```python
from build123d import *

# Parameters (mm, degrees)
IZIM1_R                     = 65
IZIM1_W                     = 20
IZIM1_H                     = 5
Y_KSEKLIK_EKSTR_ZYON1_DEPTH = 3
Y_KSEKLIK_EKSTR_ZYON2_START = 2
IZIM2_R                     = 65
Y_KSEKLIK_EKSTR_ZYON2_DEPTH = 2
SKETCH1_OUTSIDE_W           = 168.784
SKETCH1_OUTSIDE_H           = 168.784
CUT_EXTRUDE1_DEPTH          = 10


with BuildPart() as part:
    # Çizim1 → Yükseklik-Ekstrüzyon1 (new body)
    with BuildSketch(Plane.XY):
        Circle(IZIM1_R)
        Polygon((6.197521384, -35.508725619), (5.430030224, -40.449470231), (25.193008671, -43.519434871), (25.960499832, -38.578690259), (16.079010608, -37.043707939), align=None, mode=Mode.SUBTRACT)
        Polygon((8.806991329, -18.710193939), (8.039500168, -23.650938551), (17.920989392, -25.185920871), (27.802478616, -26.720903191), (28.569969776, -21.780158579), align=None, mode=Mode.SUBTRACT)
        with Locations((-33, -8.5)):
            Rectangle(IZIM1_W, IZIM1_H, mode=Mode.SUBTRACT)
        with Locations((-33, 8.5)):
            Rectangle(IZIM1_W, IZIM1_H, mode=Mode.SUBTRACT)
        Polygon((17.920989392, 25.185920871), (8.039500168, 23.650938551), (8.806991329, 18.710193939), (28.569969776, 21.780158579), (27.802478616, 26.720903191), align=None, mode=Mode.SUBTRACT)
        Polygon((16.079010608, 37.043707939), (25.960499832, 38.578690259), (25.193008671, 43.519434871), (5.430030224, 40.449470231), (6.197521384, 35.508725619), align=None, mode=Mode.SUBTRACT)
    extrude(amount=Y_KSEKLIK_EKSTR_ZYON1_DEPTH)

    # Çizim2 → Yükseklik-Ekstrüzyon2 (add)
    with BuildSketch(Plane(origin=(0, 0, 0), x_dir=(-1, 0, 0), z_dir=(0, 0, -1)).offset(Y_KSEKLIK_EKSTR_ZYON2_START)):
        Circle(IZIM2_R)
    extrude(amount=-Y_KSEKLIK_EKSTR_ZYON2_DEPTH)

    # Sketch1 outside → Cut-Extrude1 (cut)
    with BuildSketch(Plane.XY.offset(3)):
        Rectangle(SKETCH1_OUTSIDE_W, SKETCH1_OUTSIDE_H)
        with BuildLine():
            Line((-46.208680474, -21.225709885), (3.791319526, -52.34052429))
            ThreePointArc((3.791319526, -52.34052429), (29.140489861, -52.969070419), (42, -31.114814405))
            Line((42, -31.114814405), (42, 31.114814405))
            ThreePointArc((42, 31.114814405), (29.140489861, 52.969070419), (3.791319526, 52.34052429))
            Line((3.791319526, 52.34052429), (-46.208680474, 21.225709885))
            ThreePointArc((-46.208680474, 21.225709885), (-58, 0), (-46.208680474, -21.225709885))
        make_face(mode=Mode.SUBTRACT)
    extrude(amount=-CUT_EXTRUDE1_DEPTH, mode=Mode.SUBTRACT)


solid = part.part
```
Build history of the part. All positions in model axes, mm. A direction names the side the tool comes from. Round coordinates to 2 decimals unless told otherwise and drop trailing zeros. Loops run counter-clockwise (first coordinate to the right, second up) from the corner with the lowest first, then second, coordinate; pieces in that order, holes last. Notation, with made-up numbers: M 4.5,-33.5 L 43.5,-33.5 A16 cw 43.5,-7.5 Z; hole C -40,56 d3. An arc over 180 degrees is marked long. Answer as CSV lines item,"result".
1. Cut at B-B on x = -27. Write the cut outline in (y, z).
Resolved:
outline,"M -33.18,-2 L 33.18,-2 L 33.18,3 L 11,3 L 11,0 L 6,0 L 6,3 L -6,3 L -6,0 L -11,0 L -11,3 L -33.18,3 Z"
2. Flat gauge pins, fed straight in: P1, Ø1.5, axis at y = -8.5, z = 1.5, coming from the -X side; P2, Ø1.5, axis at y = 34.5, z = 0.5, coming from the -X side; P3, Ø2.5, axis at x = -28.5, y = -8, coming from the +Z side. Where does each tip first touch, or does it go through?
Resolved:
P1,"stops at x = -56.77"
P2,"stops at x = -26.08"
P3,"stops at z = 0"
3. Cut at C-C on y = -32.5. Write the cut outline in (x, z).
Resolved:
outline,"M -28.09,-2 L 41.96,-2 L 41.96,3 L -28.09,3 Z"
4. Wall check: probe 1 along Y at (x, z) = (24, 0.65); probe 2 along Z at (x, y) = (12, -19.5); probe 3 along Y at (x, z) = (26, 1.75). Give the ranges that are in metal, low to high. Write a range as [from, to].
Resolved:
probe 1,"y = [-55.11, -43.33], [-38.27, -26.13], [-21.07, 21.07], [26.13, 38.27], [43.33, 55.11]"
probe 2,"z = [-2, 0]"
probe 3,"y = [-54.44, -26.44], [-21.38, 21.38], [26.44, 54.44]"
5. 3-axis set-ups, long thin cutter, end or side, ignore diameter. For faces 1 (the flat face through (42, 0, 1)), 2 (the flat face through (16, -39, 0)): which of +Z, -Z, +X, -X, +Y, -Y reach the whole face in a straight line?
Resolved:
face 1,"+Z, -Z, +X, +Y, -Y"
face 2,"+Z"
6. Cut at A-A on z = 1. Count the separate pieces of the cut face and the enclosed holes in it, then the cut area to 3 significant figures.
Resolved:
separate pieces,"1"
enclosed holes,"6"
area,"7,420 mm²"
7. Cut at D-D on x = 22. Write the cut outline in (y, z).
Resolved:
outline,"M -55.61,-2 L 55.61,-2 L 55.61,3 L 43.02,3 L 43.02,0 L 37.96,0 L 37.96,3 L 25.82,3 L 25.82,0 L 20.76,0 L 20.76,3 L -20.76,3 L -20.76,0 L -25.82,0 L -25.82,3 L -37.96,3 L -37.96,0 L -43.02,0 L -43.02,3 L -55.61,3 Z"
8. Two-plate mould, pull along X, no slides. Class faces 3 (the flat face through (2, 1, 3)), 4 (the flat face through (-43, -9, 1)), 5 (the cylindrical face through (28.81, -53.15, 0.54)): released by +X, released by -X, zero draft, split by the parting line, or undercut.
Resolved:
face 3,"zero draft"
face 4,"undercut"
face 5,"split by the parting line"
